```python
from build123d import *

# Parameters (mm, degrees)
F0_W     = 203.2
F0_H     = 53.975
F1_DEPTH = 4.7625
F2_SIZE  = 8.636
F3_W     = 203.2
F3_H     = 19.05
F4_DEPTH = 6.35


with BuildPart() as f1:
    # F0 (on Front) → F1 (new body, symmetric)
    with BuildSketch(Plane.XZ):
        Rectangle(F0_W, F0_H)
    extrude(amount=F1_DEPTH, both=True)

    # F2
    f2_edges = [f1.edges().sort_by_distance(p)[0] for p in [
        (0, -4.7625, 26.9875),
        (0, -4.7625, -26.9875),
    ]]
    chamfer(f2_edges, length=F2_SIZE)

    # F3 (on face) → F4 (join)
    with BuildSketch(Plane.XZ.offset(4.7625)):
        Rectangle(F3_W, F3_H)
    extrude(amount=F4_DEPTH)


solid = f1.part
```
CAD build for the part. Positions are in the model's coordinates, mm. A direction names the side the tool comes from. Coordinates: 2 decimals unless noted, no trailing zeros. Order: outer loops, then holes, each group sorted by start corner. A loop starts at its lowest first (then second) coordinate and runs counter-clockwise, first axis right, second up. Notation, with made-up numbers: M 60,-3 L 69,-3 A10 ccw 69,2 Z; hole C -39.75,83.25 d3. An arc over 180 degrees is marked long. Write each question's results on one line, items separated by ' | '. Start each with the question number.
Q1. Cut at A-A (x = 83). List the corners of the cut face in (y, z) (1 decimal), then the cut area to 4 significant figures.
Q2. Which spindle directions (+Z, -Z, +X, -X, +Y, -Y) get a long thin tool onto all of the face, cutting with end or side? Do faces 1 (the flat face through (-1, -11.112, 0)), 2 (the flat face through (-1, -4.762, -14)), 3 (the flat face through (-1, -4.762, 14)). Say none if no direction does.
Q3. Cut at B-B (z = 16.5). List the corners of the cut face in (x, y), then the cut area to 3 significant figures.
Q4. Drill centre lines: probe 1 along Z at (x, y) = (74, -10.25) (3 decimals); probe 2 along Y at (x, z) = (8, 11); probe 3 along Y at (x, z) = (5.5, 23). Where is each one in solid material? Low to high. Write a range as from..to.
Q5. Cut at C-C (y = -7.75). List the corners of the cut face in (x, z) (3 decimals), then the cut area to 3 significant figures.
Q6. Flat gauge pins, fed straight in: P1, Ø5, axis at x = 12.5, y = -8, coming from the +Z side (3 decimals); P2, Ø3, axis at x = -23.5, y = -7.5, coming from the -Z side (3 decimals); P3, Ø10, axis at x = 53, z = -21.5, coming from the -Y side. Where does each tip first touch, or does it go through?
Found:
1) outline: M -11.1,-9.5 L -4.8,-9.5 L -4.8,-18.4 L 3.9,-27 L 4.8,-27 L 4.8,27 L 3.9,27 L -4.8,18.4 L -4.8,9.5 L -11.1,9.5 Z | area: 560.5 mm²
2) face 1: +Z, -Z, +X, -X, -Y | face 2: -Z, +X, -X, -Y | face 3: +Z, +X, -X, -Y
3) outline: M -101.6,-4.76 L 101.6,-4.76 L 101.6,4.76 L -101.6,4.76 Z | area: 1,940 mm²
4) probe 1: -9.525..9.525 | probe 2: -4.76..4.76 | probe 3: -0.11..4.76
5) outline: M -101.6,-9.525 L 101.6,-9.525 L 101.6,9.525 L -101.6,9.525 Z | area: 3,870 mm²
6) P1: z = 9.525 | P2: z = -9.525 | P3: y = -4.76
